Geometry check sheet. Reference: the model listing, model coordinates, mm. A direction names the side the tool comes from. Round coordinates to 2 decimals unless told otherwise and drop trailing zeros. Order: outer loops, then holes, each group sorted by start corner. A loop starts at its lowest first (then second) coordinate and runs counter-clockwise, first axis right, second up.
```python
from build123d import *

# Parameters (mm, degrees)
BOSS_EXTRUDE1_DEPTH = 5.6
SKETCH2_R           = 1.7
CUT_EXTRUDE1_DEPTH  = 16.9
CUT_EXTRUDE2_DEPTH  = 2.4


with BuildPart() as part:
    # Sketch1 → Boss-Extrude1 (new body)
    with BuildSketch(Plane(origin=(0, 0, 0), x_dir=(1, 0, 0), z_dir=(0, 1, 0))):
        with BuildLine():
            Line((-7.95, -20), (-7.95, 0))
            ThreePointArc((-7.95, 0), (0, 7.95), (7.95, 0))
            Line((7.95, 0), (7.95, -20))
            Line((7.95, -20), (0.75, -20))
            Line((0.75, -20), (0.75, -3.979949748))
            ThreePointArc((0.75, -3.979949748), (0, 4.05), (-0.75, -3.979949748))
            Line((-0.75, -3.979949748), (-0.75, -20))
            Line((-0.75, -20), (-7.95, -20))
        make_face()
    extrude(amount=BOSS_EXTRUDE1_DEPTH)

    # Sketch2 → Cut-Extrude1 (cut, through all)
    with BuildSketch(Plane.ZY.offset(7.95)):
        with Locations((14, 2.8)):
            Circle(SKETCH2_R)
    extrude(amount=-CUT_EXTRUDE1_DEPTH, mode=Mode.SUBTRACT)

    # Sketch4 → Cut-Extrude2 (cut)
    with BuildSketch(Plane(origin=(7.95, 0, 0), x_dir=(0, 0, -1), z_dir=(1, 0, 0))):
        Polygon((-17.464101615, 2.8), (-15.847520861, 5.6), (-12.152479139, 5.6), (-10.535898385, 2.8), (-12.152479139, 0), (-15.847520861, 0), align=None)
    extrude(amount=-CUT_EXTRUDE2_DEPTH, mode=Mode.SUBTRACT)


solid = part.part
```
(1) Sectioned sample at D-D, the plane x = 2.75. Record the cut outline in (y, z), and give its area (3 significant figures).
Returned:
outline: (0, -7.46) - (5.6, -7.46) - (5.6, -2.97) - (0, -2.97) - close; (0, 2.97) - (5.6, 2.97) - (5.6, 20) - (0, 20) - close; hole circle Ø3.4 at (2.8, 14)
area: 111 mm2
(2) Material ranges on line 1 (X direction, y = 0.6, z = 11); line 2 (Z direction, x = -2, y = 1.3); line 3 (Z direction, x = 3.25, y = 3.4), recorded low to high.
Returned:
line 1: x = -7.95 to -0.75, 0.75 to 7.95
line 2: z = -7.69 to -3.52, 3.52 to 13.2, 14.8 to 20
line 3: z = -7.26 to -2.42, 2.42 to 12.41, 15.59 to 20
(3) Sectioned sample at B-B, the plane z = 14. Record the cut outline in (x, y).
Returned:
outline: (-7.95, 0) - (-0.75, 0) - (-0.75, 1.1) - (-7.95, 1.1) - close; (-7.95, 4.5) - (-0.75, 4.5) - (-0.75, 5.6) - (-7.95, 5.6) - close; (0.75, 0) - (5.55, 0) - (5.55, 1.1) - (0.75, 1.1) - close; (0.75, 4.5) - (5.55, 4.5) - (5.55, 5.6) - (0.75, 5.6) - close
(4) Sectioned sample at C-C, the plane z = 9.75. Record the cut outline in (x, y).
Returned:
outline: (-7.95, 0) - (-0.75, 0) - (-0.75, 5.6) - (-7.95, 5.6) - close; (0.75, 0) - (7.95, 0) - (7.95, 5.6) - (0.75, 5.6) - close
(5) Sectioned sample at A-A, the plane x = -1.25. Record the cut outline in (y, z).
Returned:
outline: (0, -7.85) - (5.6, -7.85) - (5.6, -3.85) - (0, -3.85) - close; (0, 3.85) - (5.6, 3.85) - (5.6, 20) - (0, 20) - close; hole circle Ø3.4 at (2.8, 14)
(6) Draft check along Z on faces 1 (the flat face through (6.767, 4.18, 16.667)), 2 (the cylindrical face through (3.12, 2.15, 15.57)), 3 (the flat face through (-4, 3, 20)), 4 (the flat face through (7.95, 3, 18)). Enter one of: released by +Z, released by -Z, zero draft, split by the parting line, or undercut.
Returned:
face 1: undercut
face 2: undercut
face 3: released by +Z
face 4: zero draft
(7) Depth check by flat-ended pin: P1, Ø3, axis at y = 2.5, z = -4.5, coming from the -X side; P2, Ø7.5, axis at x = 0, z = 0, coming from the +Y side; P3, Ø1.7, axis at y = 2, z = 12.5, coming from the +X side. Enter the tip coordinate at first touch or a pass-through.
Returned:
P1: stops at x = -7.36
P2: passes through
P3: stops at x = 5.55
(8) Set-up check for faces 5 (the flat face through (-0.75, 3, 12)), 6 (the flat face through (6.767, 1.42, 11.333)), 7 (the cylindrical face through (-4.4, 2.15, 15.57)): record each of +Z, -Z, +X, -X, +Y, -Y from which the full face is reachable in a straight line by a thin tool's end or side.
Returned:
face 5: +Z, +Y, -Y
face 6: +X
face 7: +X, -X
